For this review, take the finished solid that the model builds, in its own axes (mm). Face numbers are marked on the shaded views. Give positions to 0.01 mm unless a question says otherwise; leave off trailing zeros. Write each loop counter-clockwise with the first axis right and the second up, starting at its lowest first coordinate (ties: lowest second). Pieces come first, ordered by that corner, then holes. Notation, with made-up numbers: (-16.5, 2.25) -> (37.5, 2.25) arc R25 cw to (37.5, 33.25) -> close; hole circle Ø8 at (33, -30.75). An arc over 180 degrees is marked (long way). Return JSON: item names as keys, results as strings.
from build123d import *

# Parameters (mm, degrees)
F1_DEPTH = 25.4
F3_DEPTH = 19.05
F4_D     = 15.875
F4_DEPTH = 19.05
F4_TIP   = 4.7693311635


# Not quite as in the source:
# - a length typed as a fraction of an inch, garbled in the dataset ("3 / 203.2 mm" for 3/8 in), is restored


with BuildPart() as f1:
    # F0 (on Top) → F1 (new body)
    with BuildSketch(Plane.XY):
        with BuildLine():
            ThreePointArc((-196.85, -59.69), (-193.1302561211, -68.6702561211), (-184.15, -72.39))
            Line((-184.15, -72.39), (184.15, -72.39))
            ThreePointArc((184.15, -72.39), (193.1302561211, -68.6702561211), (196.85, -59.69))
            Line((196.85, -59.69), (196.85, 59.69))
            ThreePointArc((196.85, 59.69), (193.1302561211, 68.6702561211), (184.15, 72.39))
            Line((184.15, 72.39), (-184.15, 72.39))
            ThreePointArc((-184.15, 72.39), (-193.1302561211, 68.6702561211), (-196.85, 59.69))
            Line((-196.85, 59.69), (-196.85, -59.69))
        make_face()
    extrude(amount=-F1_DEPTH)

    # F2 (on Top) → F3 (cut)
    with BuildSketch(Plane.XY):
        with BuildLine():
            Line((22.1926261067, 13.97), (-6.35, 13.97))
            ThreePointArc((-6.35, 13.97), (-15.3302561211, 10.2502561211), (-19.05, 1.27))
            Line((-19.05, 1.27), (-19.05, -46.99))
            ThreePointArc((-19.05, -46.99), (-15.3302561211, -55.9702561211), (-6.35, -59.69))
            Line((-6.35, -59.69), (165.1, -59.69))
            ThreePointArc((165.1, -59.69), (174.0802561211, -55.9702561211), (177.8, -46.99))
            Line((177.8, -46.99), (177.8, 1.27))
            ThreePointArc((177.8, 1.27), (174.0802561211, 10.2502561211), (165.1, 13.97))
            Line((165.1, 13.97), (125.73, 13.97))
            Line((125.73, 13.97), (113.03, 13.97))
            Line((113.03, 13.97), (34.8926261067, 13.97))
            Line((34.8926261067, 13.97), (22.1926261067, 13.97))
        make_face()
        with BuildLine():
            Line((22.1926261067, 44.45), (22.1926261067, 13.97))
            Line((22.1926261067, 13.97), (34.8926261067, 13.97))
            Line((34.8926261067, 13.97), (34.8926261067, 44.45))
            ThreePointArc((34.8926261067, 44.45), (28.5426261067, 50.8), (22.1926261067, 44.45))
        make_face()
        with BuildLine():
            Line((113.03, 26.3348463923), (113.03, 13.97))
            Line((113.03, 13.97), (125.73, 13.97))
            Line((125.73, 13.97), (125.73, 26.3348463923))
            ThreePointArc((125.73, 26.3348463923), (119.38, 32.6848463923), (113.03, 26.3348463923))
        make_face()
        with BuildLine():
            ThreePointArc((-136.2642422318, 48.2357204892), (-147.6423993224, 51.8340887509), (-151.5906006098, 40.5725426972))
            Line((-151.5906006098, 40.5725426972), (-121.928781271, -5.026510451))
            ThreePointArc((-121.928781271, -5.026510451), (-110.8444944433, -8.0371380797), (-106.602422893, 2.636667341))
            Line((-106.602422893, 2.636667341), (-136.2642422318, 48.2357204892))
        make_face()
    extrude(amount=-F3_DEPTH, mode=Mode.SUBTRACT)

    # F4
    with Locations(Plane.XY):
        with Locations((-165.1, 44.45), (50.8, 44.45), (73.66, 44.45), (165.1, 44.45), (-165.1, 0), (-38.1, -43.18)):
            Hole(F4_D / 2, depth=F4_DEPTH)
            with Locations((0, 0, -(F4_DEPTH + F4_TIP / 2))):  # 118° drill point
                Cone(0, F4_D / 2, F4_TIP, mode=Mode.SUBTRACT)


solid = f1.part
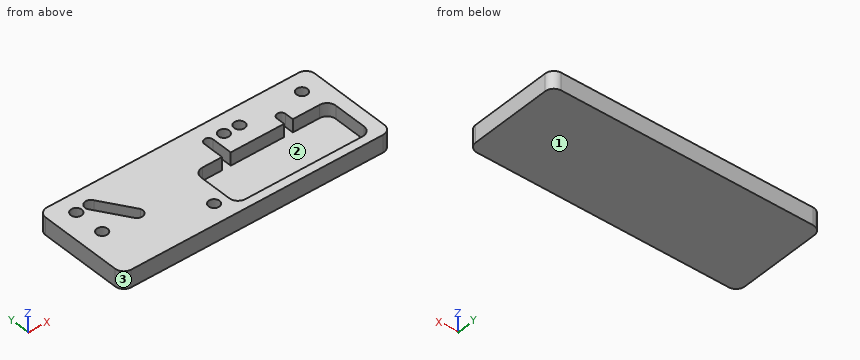
1. The part is to be moulded in two halves that separate along Y. For the marked faces 1, 2 and 3, say which applies: +Y half, -Y half, draft (parallel to the pull), parting line (faces both ways), or undercut.
Results found:
{"face 1": "draft", "face 2": "undercut", "face 3": "-Y half"}
2. Add section A-A, the plane z = -4.5. Count the separate pieces of the cut face and the enclosed holes in it, plus the area to 3 significant figures.
Results found:
{"separate pieces": "1", "enclosed holes": "8", "area": "39,500 mm²"}
3. For pin 1 (1.5 mm diameter, centred on x = 67, y = 42.5, fed in from +Z), flat-tipped, find the tip position at first contact; note if it passes through.
Results found:
{"pin 1": "stops at z = -19.2"}
4. To check wall thickness, follow probe 1 along Y at (x, z) = (-165.1, -8.5); probe 2 along Y at (x, z) = (50.8, -14); probe 3 along X at (y, z) = (-20.5, -17.5). State the ranges of each line that lie inside material, in increasing order.
Results found:
{"probe 1": "y = -72.39 to -7.94, 7.94 to 36.51, 52.39 to 72.39", "probe 2": "y = -72.39 to -59.69, 13.97 to 36.51, 52.39 to 72.39", "probe 3": "x = -196.85 to -19.05, 177.8 to 196.85"}
5. Add section B-B, the plane x = 135. State the section outline as (y, z) points.
Results found:
{"outline": "(-72.39, -25.4) -> (72.39, -25.4) -> (72.39, 0) -> (13.97, 0) -> (13.97, -19.05) -> (-59.69, -19.05) -> (-59.69, 0) -> (-72.39, 0) -> close"}
6. Add section C-C, the plane x = -110. State the section outline as (y, z) points, plus the area to 3 significant figures.
Results found:
{"outline": "(-72.39, -25.4) -> (72.39, -25.4) -> (72.39, 0) -> (7.86, 0) -> (7.86, -19.05) -> (-7.55, -19.05) -> (-7.55, 0) -> (-72.39, 0) -> close", "area": "3,380 mm²"}
